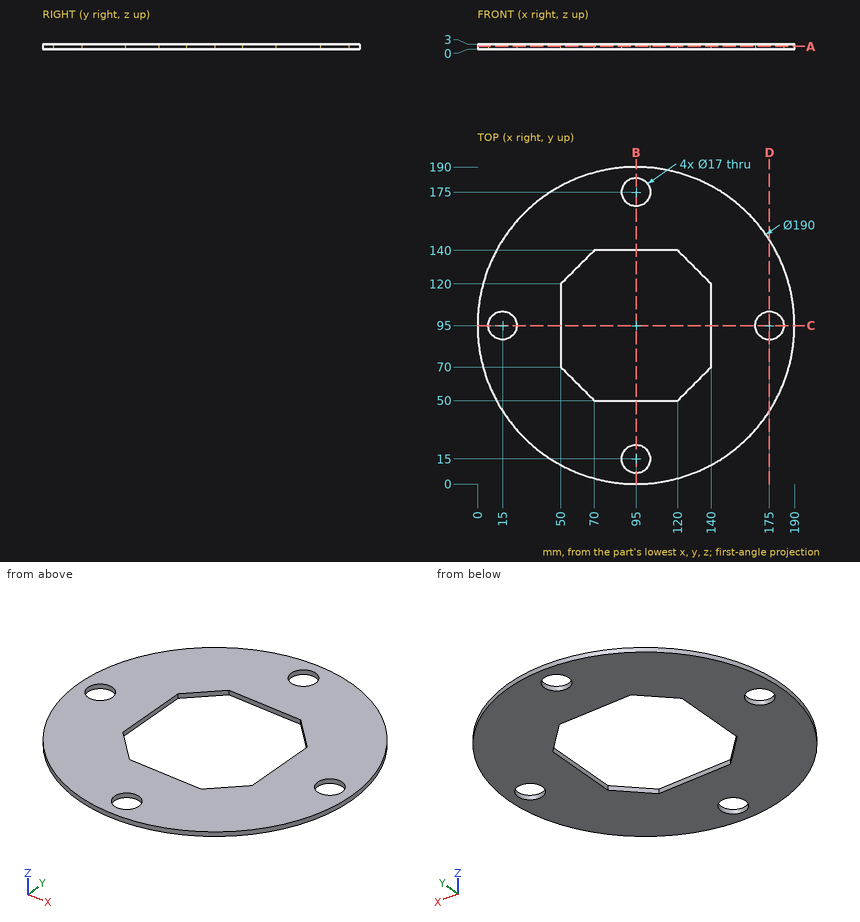
Check sheet for the drawn part. Datum: minimum x, y, z corner. Units: mm. Give positions to 0.01 mm unless a question says otherwise; leave off trailing zeros. Write each loop counter-clockwise with the first axis right and the second up, starting at its lowest first coordinate (ties: lowest second). Pieces come first, ordered by that corner, then holes.
(1) Cross-section at B-B (x = 95). Enter the section's corners in (y, z), plus the area to 3 significant figures.
(2) Material ranges on line 1 (Y direction, x = 95, z = 0.9); line 2 (Y direction, x = 90, z = 0.35); line 3 (X direction, y = 19, z = 0.95), recorded low to high.
(3) Cross-section at D-D (x = 175). Enter the section's corners in (y, z), plus the area to 3 significant figures.
(4) Cross-section at A-A (z = 1.55). Enter the section's corners in (x, y), plus the area to 3 significant figures.
(5) Gauge pin test, flat ends, axial feed: pin 1 (15.5 mm diameter, centred on x = 15, y = 95, fed in from +Z); pin 2 (1.5 mm diameter, centred on x = 91.5, z = 1, fed in from -Y); pin 3 (1.5 mm diameter, centred on y = 120, z = 2, fed in from +X); pin 4 (0.9 mm diameter, centred on x = 89.5, z = 2, fed in from +Y). Record the tip position at first contact, or that the pin passes through.
Worked out:
1. outline: (0, 0) - (6.5, 0) - (6.5, 3) - (0, 3) - close; (23.5, 0) - (50, 0) - (50, 3) - (23.5, 3) - close; (140, 0) - (166.5, 0) - (166.5, 3) - (140, 3) - close; (183.5, 0) - (190, 0) - (190, 3) - (183.5, 3) - close
1. area: 198 mm2
2. line 1: y = 0 to 6.5, 23.5 to 50, 140 to 166.5, 183.5 to 190
2. line 2: y = 0.13 to 8.13, 21.87 to 50, 140 to 168.13, 181.87 to 189.87
2. line 3: x = 38 to 87.5, 102.5 to 152
3. outline: (43.77, 0) - (86.5, 0) - (86.5, 3) - (43.77, 3) - close; (103.5, 0) - (146.23, 0) - (146.23, 3) - (103.5, 3) - close
3. area: 256 mm2
4. outline: circle Ø190 at (95, 95); hole circle Ø17 at (15, 95); hole (50, 70) - (70, 50) - (120, 50) - (140, 70) - (140, 120) - (120, 140) - (70, 140) - (50, 120) - close; hole circle Ø17 at (95, 15); hole circle Ø17 at (95, 175); hole circle Ø17 at (175, 95)
4. area: 20,100 mm2
5. pin 1: passes through
5. pin 2: stops at y = 0.04
5. pin 3: stops at x = 186.85
5. pin 4: stops at y = 189.87
